from build123d import *

# Parameters (mm, degrees)
CROQUIS1_R                   = 50
SALIENTE_EXTRUIR1_DEPTH      = 30
CROQUIS2_R                   = 45
CROQUIS2_R_2                 = 32.5
CORTAR_EXTRUIR1_DEPTH        = 2
CROQUIS3_R                   = 13
CORTAR_EXTRUIR2_DEPTH        = 6
SALIENTE_EXTRUIR2_REACH      = 144.478
SALIENTE_EXTRUIR2_END_RADIUS = 50
CROQUIS5_W                   = 60
CROQUIS5_H                   = 60
CROQUIS5_W_2                 = 50.8
CROQUIS5_H_2                 = 50.8


with BuildPart() as part:
    # Croquis1 → Saliente-Extruir1 (new, symmetric)
    with BuildSketch(Plane.XY):
        Circle(CROQUIS1_R)
    extrude(amount=SALIENTE_EXTRUIR1_DEPTH, both=True)

    # Croquis2 → Cortar-Extruir1 (cut)
    with BuildSketch(Plane(origin=(0, 0, -30), x_dir=(-1, 0, 0), z_dir=(0, 0, -1))):
        Circle(CROQUIS2_R)
        Circle(CROQUIS2_R_2, mode=Mode.SUBTRACT)
    extrude(amount=-CORTAR_EXTRUIR1_DEPTH, mode=Mode.SUBTRACT)

    # Croquis3 → Cortar-Extruir2 (cut)
    with BuildSketch(Plane(origin=(0, 0, -30), x_dir=(-1, 0, 0), z_dir=(0, 0, -1))):
        Circle(CROQUIS3_R)
    extrude(amount=-CORTAR_EXTRUIR2_DEPTH, mode=Mode.SUBTRACT)

    # Saliente-Extruir2: up to this cylinder (the profile starts outside it)
    saliente_extruir2_end = Plane(origin=(0, 0, 29.151472), z_dir=(0, 0, -1)) * Cylinder(SALIENTE_EXTRUIR2_END_RADIUS, 389.956, mode=Mode.PRIVATE)
    # Croquis5 → Saliente-Extruir2 (add, up to the surface)
    with BuildSketch(Plane(origin=(0, 80, 0), x_dir=(1, 0, 0), z_dir=(0, 1, 0)), mode=Mode.PRIVATE) as saliente_extruir2_sk1:
        Rectangle(CROQUIS5_W, CROQUIS5_H)
        Rectangle(CROQUIS5_W_2, CROQUIS5_H_2, mode=Mode.SUBTRACT)
    saliente_extruir2_tool1 = extrude(saliente_extruir2_sk1.sketch, amount=-SALIENTE_EXTRUIR2_REACH, mode=Mode.PRIVATE) - saliente_extruir2_end
    add(saliente_extruir2_tool1.solids().sort_by_distance((0, 80, 29.151472))[0])


solid = part.part
Could you check a few things on this model? Use its own coordinates, in mm. A direction names the side the tool comes from. Give positions to 0.01 mm unless a question says otherwise; leave off trailing zeros. Order: outer loops, then holes, each group sorted by start corner. A loop starts at its lowest first (then second) coordinate and runs counter-clockwise, first axis right, second up.
1. Suppose I cut it at C-C (x = 0). Write out the boundary of the cut face in (y, z), plus the area to 3 significant figures.
Answers below:
outline: (-50, -30) - (-45, -30) - (-45, -28) - (-32.5, -28) - (-32.5, -30) - (-13, -30) - (-13, -24) - (13, -24) - (13, -30) - (32.5, -30) - (32.5, -28) - (45, -28) - (45, -30) - (80, -30) - (80, -25.4) - (50, -25.4) - (50, 25.4) - (80, 25.4) - (80, 30) - (-50, 30) - close
area: 6,070 mm2
2. Thinking about a two-plate mould opening in Z: for faces 6 (the cylindrical face through (10.316, -7.91, -27.042)), 7 (the cylindrical face through (0, 50, 0)), 8 (the flat face through (-13, -30, -28)), 9 (the flat face through (-1, 16, 30)), which applies, +Z half, -Z half, draft (parallel to the pull), parting line (faces both ways), or undercut?
Answers below:
face 6: draft
face 7: undercut
face 8: -Z half
face 9: +Z half
3. Suppose I cut it at A-A (y = 58.5). Write out the boundary of the cut face in (x, z), plus the area to 3 significant figures.
Answers below:
outline: (-30, -30) - (30, -30) - (30, 30) - (-30, 30) - close; hole (-25.4, -25.4) - (25.4, -25.4) - (25.4, 25.4) - (-25.4, 25.4) - close
area: 1,020 mm2
4. Suppose I cut it at D-D (y = 0). Write out the boundary of the cut face in (x, z), plus the area to 3 significant figures.
Answers below:
outline: (-50, -30) - (-45, -30) - (-45, -28) - (-32.5, -28) - (-32.5, -30) - (-13, -30) - (-13, -24) - (13, -24) - (13, -30) - (32.5, -30) - (32.5, -28) - (45, -28) - (45, -30) - (50, -30) - (50, 30) - (-50, 30) - close
area: 5,790 mm2
5. I need wall thicknesses on L1, parallel to Y at x = 0, z = -28.75; L2, parallel to X at y = 62, z = 24; L3, parallel to Y at x = 0, z = -25.55. Which ranges of each line are inside material? Lowest first, please.
Answers below:
L1: y = -50 to -45, -32.5 to -13, 13 to 32.5, 45 to 80
L2: x = -30 to -25.4, 25.4 to 30
L3: y = -50 to -13, 13 to 80
6. Which directions (+Z, -Z, +X, -X, +Y, -Y) give clear straight access to the entire face, cutting with the end or side of a thin tool? Please do faces 1 (the flat face through (-30, 60, 0)), 2 (the flat face through (-4, 49, -30)), 3 (the flat face through (-25.4, 62, 0)), 4 (the cylindrical face through (-31, 9.76, -29.01)), 5 (the flat face through (30, 60, 0)).
Answers below:
face 1: +Z, -Z, -X, +Y
face 2: -Z, +X, -X, +Y, -Y
face 3: +Y
face 4: -Z
face 5: +Z, -Z, +X, +Y
7. For pin 1 (5 mm diameter, centred on y = 23.5, z = -5, fed in from +X); pin 2 (2 mm diameter, centred on y = -13, z = 19, fed in from -X); pin 3 (12 mm diameter, centred on y = 68, z = -10, fed in from -X), each with a flat end and sliding along its axis, tell me the tip position at first contact or that it passes through.
Answers below:
pin 1: stops at x = 45.38
pin 2: stops at x = -48.54
pin 3: stops at x = -30
8. Suppose I cut it at B-B (z = -17). Write out the boundary of the cut face in (x, y), plus the area to 3 significant figures.
Answers below:
outline: (-30, 40) arc R50 ccw (long way) to (30, 40) - (30, 80) - (25.4, 80) - (25.4, 43.07) arc R50 ccw to (-25.4, 43.07) - (-25.4, 80) - (-30, 80) - close
area: 8,210 mm2
